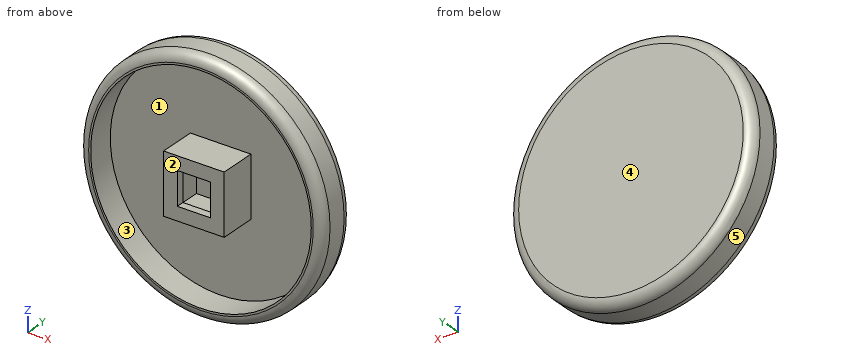
```python
from build123d import *

# Parameters (mm, degrees)
SKETCH_1_R      = 12.5
EXTRUDE_1_DEPTH = 1.2
SKETCH_1_3_R    = 12.5
SKETCH_1_3_R_2  = 11.3
EXTRUDE_2_DEPTH = 4
SKETCH_1_5_W    = 6.2
SKETCH_1_5_H    = 6.2
EXTRUDE_3_DEPTH = 2
EXTRUDE_START   = -2
SKETCH_1_6_W    = 6.2
SKETCH_1_6_H    = 6.2
SKETCH_1_6_W_2  = 3.8
SKETCH_1_6_H_2  = 3.8
EXTRUDE_4_DEPTH = 3
FILLET_1_R      = 1
SKETCH_2_W      = 3.8
SKETCH_2_H      = 3.8
SKETCH_2_W_2    = 3.4
SKETCH_2_H_2    = 3.4
EXTRUDE_5_DEPTH = 0.8


with BuildPart() as part:
    # Эскиз1 → Бобышка-Вытянуть1 (new body)
    with BuildSketch(Plane(origin=(0, 0, 0), x_dir=(1, 0, 0), z_dir=(0, 1, 0))):
        Circle(SKETCH_1_R)
    extrude(amount=-EXTRUDE_1_DEPTH)

    # Эскиз1<3> → Бобышка-Вытянуть2 (add)
    with BuildSketch(Plane(origin=(0, 0, 0), x_dir=(1, 0, 0), z_dir=(0, 1, 0))):
        Circle(SKETCH_1_3_R)
        Circle(SKETCH_1_3_R_2, mode=Mode.SUBTRACT)
    extrude(amount=-EXTRUDE_2_DEPTH)

    # Эскиз1<5> → Бобышка-Вытянуть3 (add)
    with BuildSketch(Plane(origin=(0, 0, 0), x_dir=(1, 0, 0), z_dir=(0, 1, 0))):
        Rectangle(SKETCH_1_5_W, SKETCH_1_5_H)
    extrude(amount=-EXTRUDE_3_DEPTH)

    # Эскиз1<6> → Бобышка-Вытянуть4 (add)
    with BuildSketch(Plane(origin=(0, 0, 0), x_dir=(1, 0, 0), z_dir=(0, 1, 0)).offset(EXTRUDE_START)):
        Rectangle(SKETCH_1_6_W, SKETCH_1_6_H)
        Rectangle(SKETCH_1_6_W_2, SKETCH_1_6_H_2, mode=Mode.SUBTRACT)
    extrude(amount=-EXTRUDE_4_DEPTH)

    # Скругление1
    fillet_1_edges = [part.edges().sort_by_distance(p)[0] for p in [
        (-12.5, 0, 0),
        (-12.5, -4, 0),
    ]]
    fillet(fillet_1_edges, radius=FILLET_1_R)

    # Эскиз2 → Бобышка-Вытянуть5 (add)
    with BuildSketch(Plane.XZ.offset(5)):
        Rectangle(SKETCH_2_W, SKETCH_2_H)
        Rectangle(SKETCH_2_W_2, SKETCH_2_H_2, mode=Mode.SUBTRACT)
    extrude(amount=-EXTRUDE_5_DEPTH)


solid = part.part
```
Work out the finished part from the listing and answer in its coordinate system (mm). Face numbers are marked on the shaded views. A direction names the side the tool comes from. Coordinates: 2 decimals unless noted, no trailing zeros. Loops run counter-clockwise (first coordinate to the right, second up) from the corner with the lowest first, then second, coordinate; pieces in that order, holes last. Notation, with made-up numbers: (30.25, 8) - (68.25, 8) arc R28 ccw to (68.25, 41) - close; hole circle Ø8 at (0.25, 13.25). An arc over 180 degrees is marked (long way). Use a Markdown table: item, result.
Item 1: Find section B-B, the plane x = 0. Determine the outline of the cut face in (y, z).
Evaluation:
| item | result |
|---|---|
| outline | (-5, -3.1) - (-1.2, -3.1) - (-1.2, -11.3) - (-4, -11.3) - (-4, -11.5) arc R1 ccw to (-3, -12.5) - (-1, -12.5) arc R1 ccw to (0, -11.5) - (0, 11.5) arc R1 ccw to (-1, 12.5) - (-3, 12.5) arc R1 ccw to (-4, 11.5) - (-4, 11.3) - (-1.2, 11.3) - (-1.2, 3.1) - (-5, 3.1) - (-5, 1.7) - (-4.2, 1.7) - (-4.2, 1.9) - (-2, 1.9) - (-2, -1.9) - (-4.2, -1.9) - (-4.2, -1.7) - (-5, -1.7) - close |
Item 2: Find section C-C, the plane z = 0. Determine the outline of the cut face in (x, y), and give its area (3 significant figures).
Evaluation:
| item | result |
|---|---|
| outline | (-12.5, -3) arc R1 ccw to (-11.5, -4) - (-11.3, -4) - (-11.3, -1.2) - (-3.1, -1.2) - (-3.1, -5) - (-1.7, -5) - (-1.7, -4.2) - (-1.9, -4.2) - (-1.9, -2) - (1.9, -2) - (1.9, -4.2) - (1.7, -4.2) - (1.7, -5) - (3.1, -5) - (3.1, -1.2) - (11.3, -1.2) - (11.3, -4) - (11.5, -4) arc R1 ccw to (12.5, -3) - (12.5, -1) arc R1 ccw to (11.5, 0) - (-11.5, 0) arc R1 ccw to (-12.5, -1) - close |
| area | 48.3 mm2 |
Item 3: For the marked faces 1 and 2, determine the directions among +Z, -Z, +X, -X, +Y, -Y from which every point of the face is accessible in a straight line to the end or side of a thin tool.
Evaluation:
| item | result |
|---|---|
| face 1 | -Y |
| face 2 | +Z, -Z, +X, -X, -Y |
Item 4: Consider probe 1 along X at (y, z) = (-2.65, 0); probe 2 along X at (y, z) = (-2.95, 2). Determine where each line is inside the solid, lowest interval first. Write a range as from..to.
Evaluation:
| item | result |
|---|---|
| probe 1 | x = -12.5..-11.3, -3.1..-1.9, 1.9..3.1, 11.3..12.5 |
| probe 2 | x = -12.34..-11.12, -3.1..3.1, 11.12..12.34 |
Item 5: Find section D-D, the plane y = -0.4. Determine the outline of the cut face in (x, z).
Evaluation:
| item | result |
|---|---|
| outline | circle Ø24.6 at (0, 0) |
Item 6: Find section A-A, the plane y = -2.55. Determine the outline of the cut face in (x, z), and give its area (3 significant figures).
Evaluation:
| item | result |
|---|---|
| outline | circle Ø25 at (0, 0); (-3.1, -3.1) - (3.1, -3.1) - (3.1, 3.1) - (-3.1, 3.1) - close; hole circle Ø22.6 at (0, 0); hole (-1.9, -1.9) - (1.9, -1.9) - (1.9, 1.9) - (-1.9, 1.9) - close |
| area | 114 mm2 |
Item 7: The mould has two halves that part along X. Classify the marked faces 3, 4 and 5: +X half, -X half, draft (parallel to the pull), parting line (faces both ways), or undercut.
Evaluation:
| item | result |
|---|---|
| face 3 | undercut |
| face 4 | draft |
| face 5 | parting line |
Item 8: Given pin 1 Ø12 at (x, z) = (-4, -6.5) entering from -Y; pin 2 Ø1 at (x, z) = (-9.5, 4.5) entering from -Y; pin 3 Ø0.6 at (x, y) = (-0.5, -4.5) entering from -Z, each flat-ended and moving along its own axis, determine where each tip first touches the part or whether it passes through.
Evaluation:
| item | result |
|---|---|
| pin 1 | stops at y = -5 |
| pin 2 | stops at y = -1.2 |
| pin 3 | stops at z = -3.1 |
